```python
from build123d import *

# Parameters (mm, degrees)
SKETCH1_W                 = 80
SKETCH1_H                 = 50
SKETCH1_R                 = 5.588
SKETCH1_R_2               = 2.6
BOSS_EXTRUDE1_DEPTH       = 12
SKETCH2_R                 = 4.6
CUT_EXTRUDE1_DEPTH        = 1.55
M5X0_8_TAPPED_HOLE1_D     = 4.2
M5X0_8_TAPPED_HOLE2_D     = 4.2
M5X0_8_TAPPED_HOLE2_DEPTH = 14
M5X0_8_TAPPED_HOLE2_TIP   = 1.2618073
SKETCH7_R                 = 8.05
CUT_EXTRUDE2_DEPTH        = 4.5


with BuildPart() as part:
    # Sketch1 → Boss-Extrude1 (new body)
    with BuildSketch(Plane.XY):
        with Locations((40, 25)):
            Rectangle(SKETCH1_W, SKETCH1_H)
        with Locations((40, 32.4)):
            Circle(SKETCH1_R, mode=Mode.SUBTRACT)
        with Locations((30, 10)):
            Circle(SKETCH1_R_2, mode=Mode.SUBTRACT)
        with Locations((10, 30)):
            Circle(SKETCH1_R_2, mode=Mode.SUBTRACT)
        with Locations((50, 10)):
            Circle(SKETCH1_R_2, mode=Mode.SUBTRACT)
        with Locations((70, 30)):
            Circle(SKETCH1_R_2, mode=Mode.SUBTRACT)
    extrude(amount=BOSS_EXTRUDE1_DEPTH)

    # Sketch2 → Cut-Extrude1 (cut)
    with BuildSketch(Plane.XY.offset(12)):
        with Locations((10, 30)):
            Circle(SKETCH2_R)
        with Locations((30, 10)):
            Circle(SKETCH2_R)
        with Locations((50, 10)):
            Circle(SKETCH2_R)
        with Locations((70, 30)):
            Circle(SKETCH2_R)
    extrude(amount=-CUT_EXTRUDE1_DEPTH, mode=Mode.SUBTRACT)

    # M5x0.8 Tapped Hole1 (through all)
    with Locations(Plane.XY.offset(12)):
        with Locations((16.43, 8.9), (63.57, 8.9)):
            Hole(M5X0_8_TAPPED_HOLE1_D / 2)

    # M5x0.8 Tapped Hole2
    with Locations(Plane(origin=(0, 50, 0), x_dir=(1, 0, 0), z_dir=(0, 1, 0))):
        with Locations((30, -6), (50, -6)):
            Hole(M5X0_8_TAPPED_HOLE2_D / 2, depth=M5X0_8_TAPPED_HOLE2_DEPTH)
            with Locations((0, 0, -(M5X0_8_TAPPED_HOLE2_DEPTH + M5X0_8_TAPPED_HOLE2_TIP / 2))):  # 118° drill point
                Cone(0, M5X0_8_TAPPED_HOLE2_D / 2, M5X0_8_TAPPED_HOLE2_TIP, mode=Mode.SUBTRACT)

    # Sketch7 → Cut-Extrude2 (cut)
    with BuildSketch(Plane(origin=(0, 0, 0), x_dir=(-1, 0, 0), z_dir=(0, 0, -1))):
        with Locations((-40, 32.4)):
            Circle(SKETCH7_R)
    extrude(amount=-CUT_EXTRUDE2_DEPTH, mode=Mode.SUBTRACT)


solid = part.part
```
Model file for the job. Use its own axes, mm. A direction names the side the tool comes from. Coordinates: 2 decimals unless noted, no trailing zeros. Loops run counter-clockwise (first coordinate to the right, second up) from the corner with the lowest first, then second, coordinate; pieces in that order, holes last. Notation, with made-up numbers: (58, 14) -> (107, 14) arc R24 ccw to (107, 40) -> close; hole circle Ø7 at (21, 64). An arc over 180 degrees is marked (long way). Answer as a JSON object with one key per item and string values.
Q1. Cut at A-A (x = 63.57). List the corners of the cut face in (y, z), and give its area (3 significant figures).
Report:
{"outline": "(0, 0) -> (6.8, 0) -> (6.8, 12) -> (0, 12) -> close; (11, 0) -> (50, 0) -> (50, 12) -> (11, 12) -> close", "area": "550 mm2"}
Q2. Cut at C-C (y = 30). List the corners of the cut face in (x, z).
Report:
{"outline": "(0, 0) -> (7.4, 0) -> (7.4, 10.45) -> (5.4, 10.45) -> (5.4, 12) -> (0, 12) -> close; (12.6, 0) -> (32.32, 0) -> (32.32, 4.5) -> (34.95, 4.5) -> (34.95, 12) -> (14.6, 12) -> (14.6, 10.45) -> (12.6, 10.45) -> close; (45.05, 4.5) -> (47.68, 4.5) -> (47.68, 0) -> (67.4, 0) -> (67.4, 10.45) -> (65.4, 10.45) -> (65.4, 12) -> (45.05, 12) -> close; (72.6, 0) -> (80, 0) -> (80, 12) -> (74.6, 12) -> (74.6, 10.45) -> (72.6, 10.45) -> close"}
Q3. Cut at B-B (z = 9). List the corners of the cut face in (x, y), and give its area (3 significant figures).
Report:
{"outline": "(0, 0) -> (80, 0) -> (80, 50) -> (0, 50) -> close; hole circle Ø5.2 at (10, 30); hole circle Ø4.2 at (16.43, 8.9); hole circle Ø5.2 at (30, 10); hole circle Ø11.18 at (40, 32.4); hole circle Ø5.2 at (50, 10); hole circle Ø4.2 at (63.57, 8.9); hole circle Ø5.2 at (70, 30)", "area": "3,790 mm2"}
Q4. Cut at D-D (x = 40). List the corners of the cut face in (y, z).
Report:
{"outline": "(0, 0) -> (24.35, 0) -> (24.35, 4.5) -> (26.81, 4.5) -> (26.81, 12) -> (0, 12) -> close; (37.99, 4.5) -> (40.45, 4.5) -> (40.45, 0) -> (50, 0) -> (50, 12) -> (37.99, 12) -> close"}
Q5. Flat gauge pin, fed straight in: P1, Ø7.5, axis at x = 10, y = 30, coming from the +Z side. Where does the tip first touch, or does it go through?
Report:
{"P1": "stops at z = 10.45"}
Q6. Probe probe 1 along X at (y, z) = (40, 5.75); probe 2 along Y at (x, z) = (63.57, 6); probe 3 along Y at (x, z) = (50, 2.75). List the from-to ranges inside material, lowest first.
Report:
{"probe 1": "x = 0 to 27.91, 32.09 to 47.91, 52.09 to 80", "probe 2": "y = 0 to 6.8, 11 to 50", "probe 3": "y = 0 to 7.4, 12.6 to 50"}
Q7. Pull direction X, two halves, no side cores. Call faces 4 (the flat face through (80, 25, 6)), 5 (the flat face through (39, 25, 12)), 6 (the conical face through (30.2, 34.96, 5.69)): released by +X, released by -X, zero draft, split by the parting line, or undercut.
Report:
{"face 4": "released by +X", "face 5": "zero draft", "face 6": "undercut"}
Q8. 3-axis set-ups, long thin cutter, end or side, ignore diameter. For faces 1 (the cylindrical face through (48.042, 32.754, 2.218)), 2 (the cylindrical face through (14.25, 28.24, 11.24)), 3 (the conical face through (50.35, 34.96, 5.89)): which of +Z, -Z, +X, -X, +Y, -Y reach the whole face in a straight line?
Report:
{"face 1": "-Z", "face 2": "+Z", "face 3": "+Y"}
